from build123d import *

# Parameters (mm, degrees)
SKETCH_1_R          = 2.05
SKETCH_1_R_2        = 11.5
SKETCH_1_R_3        = 1.5
SKETCH_1_R_4        = 7.02
SKETCH_1_W          = 2.1
SKETCH_1_H          = 8.1
EXTRUDE_1_DEPTH     = 2
SKETCH_2_R          = 2
CUT_EXTRUDE_1_DEPTH = 4
FILLET_1_R          = 2


with BuildPart() as part:
    # 草图1 → 凸台-拉伸1 (new body)
    with BuildSketch(Plane.XY):
        with BuildLine():
            Line((-4.357142857, -0.045714286), (-4.357142857, 41.804285714))
            Line((-4.357142857, 41.804285714), (8.642857143, 41.804285714))
            Line((8.642857143, 41.804285714), (8.642857143, 14.954285714))
            Line((8.642857143, 14.954285714), (17.642857143, 14.954285714))
            Line((17.642857143, 14.954285714), (17.642857143, 41.804285714))
            Line((17.642857143, 41.804285714), (200.642857143, 41.804285714))
            Line((200.642857143, 41.804285714), (231.642857143, 30.954285714))
            ThreePointArc((231.642857143, 30.954285714), (262.642857143, -0.045714286), (231.642857143, -31.045714286))
            Line((231.642857143, -31.045714286), (200.656073527, -36.45591431))
            Line((200.656073527, -36.45591431), (193.846868021, -38.045714286))
            Line((193.846868021, -38.045714286), (22.465844759, -38.045714286))
            Line((22.465844759, -38.045714286), (3.792857143, -38.195714286))
            Line((3.792857143, -38.195714286), (3.792857143, -35.702553436))
            Line((3.792857143, -35.702553436), (-4.357142857, -35.702553436))
            Line((-4.357142857, -35.702553436), (-4.357142857, -0.045714286))
        make_face()
        with Locations((1.642857143, 29.954285714)):
            Circle(SKETCH_1_R, mode=Mode.SUBTRACT)
        with Locations((1.642857143, -0.045714286)):
            Circle(SKETCH_1_R, mode=Mode.SUBTRACT)
        with Locations((1.642857143, -30.045714286)):
            Circle(SKETCH_1_R, mode=Mode.SUBTRACT)
        with Locations((51.642857143, -0.045714286)):
            Circle(SKETCH_1_R_2, mode=Mode.SUBTRACT)
        with Locations((51.642857143, -14.045714286)):
            Circle(SKETCH_1_R_3, mode=Mode.SUBTRACT)
        with Locations((37.642857143, -0.045714286)):
            Circle(SKETCH_1_R_3, mode=Mode.SUBTRACT)
        with Locations((51.642857143, 13.954285714)):
            Circle(SKETCH_1_R_3, mode=Mode.SUBTRACT)
        with Locations((65.642857143, -0.045714286)):
            Circle(SKETCH_1_R_3, mode=Mode.SUBTRACT)
        with Locations((231.642857143, -0.045714286)):
            Circle(SKETCH_1_R_4, mode=Mode.SUBTRACT)
        with Locations((1.642857143, 14.954285714)):
            Rectangle(SKETCH_1_W, SKETCH_1_H, mode=Mode.SUBTRACT)
        with Locations((1.642857143, -15.045714286)):
            Rectangle(SKETCH_1_W, SKETCH_1_H, mode=Mode.SUBTRACT)
    extrude(amount=EXTRUDE_1_DEPTH)

    # 草图2 → 切除-拉伸1 (cut)
    with BuildSketch(Plane.XY.offset(2)):
        with Locations((26.642857143, 35.754285714)):
            Circle(SKETCH_2_R)
        with Locations((111.642857143, 35.754285714)):
            Circle(SKETCH_2_R)
        with Locations((196.642857143, 35.754285714)):
            Circle(SKETCH_2_R)
        with Locations((111.642857143, -34.245714286)):
            Circle(SKETCH_2_R)
        with Locations((196.642857143, -34.245714286)):
            Circle(SKETCH_2_R)
        with Locations((26.642857143, -34.245714286)):
            Circle(SKETCH_2_R)
        Polygon((187.542857143, -24.245714286), (140.41622539, -24.245714286), (187.542857143, 14.56445304), align=None)
        Polygon((122.542857143, 25.754285714), (169.669488896, 25.754285714), (122.542857143, -13.055881612), align=None)
        with BuildLine():
            Line((72.808867631, 8.954285714), (102.642857143, 8.954285714))
            Line((102.642857143, 8.954285714), (102.642857143, 26.754285714))
            Line((102.642857143, 26.754285714), (50.657939371, 26.754285714))
            Line((50.657939371, 26.754285714), (55.363054959, 22.651424922))
            ThreePointArc((55.363054959, 22.651424922), (65.846157695, 18.044787461), (72.808867631, 8.954285714))
        make_face()
        with BuildLine():
            Line((102.642857143, -9.045714286), (102.642857143, -26.845714286))
            Line((102.642857143, -26.845714286), (50.657939371, -26.845714286))
            Line((50.657939371, -26.845714286), (55.363054959, -22.742853493))
            ThreePointArc((55.363054959, -22.742853493), (65.846157695, -18.136216032), (72.808867631, -9.045714286))
            Line((72.808867631, -9.045714286), (102.642857143, -9.045714286))
        make_face()
        with BuildLine():
            Line((125.279005787, -19.870759717), (160.01586639, 8.736066661))
            ThreePointArc((160.01586639, 8.736066661), (163.433418031, 8.405335857), (163.102687227, 4.987784217))
            Line((163.102687227, 4.987784217), (128.365826624, -23.619042162))
            ThreePointArc((128.365826624, -23.619042162), (124.948274984, -23.288311358), (125.279005787, -19.870759717))
        make_face()
    extrude(amount=-CUT_EXTRUDE_1_DEPTH, mode=Mode.SUBTRACT)

    # 圆角1
    fillet_1_edges = [part.edges().sort_by_distance(p)[0] for p in [
        (72.808867631, 8.954285714, 1),
        (50.657939371, 26.754285714, 1),
        (102.642857143, 26.754285714, 1),
        (122.542857143, -13.055881612, 1),
        (122.542857143, 25.754285714, 1),
        (169.669488896, 25.754285714, 1),
        (187.542857143, 14.56445304, 1),
        (187.542857143, -24.245714286, 1),
        (140.41622539, -24.245714286, 1),
        (102.642857143, -26.845714286, 1),
        (50.657939371, -26.845714286, 1),
        (72.808867631, -9.045714286, 1),
        (102.642857143, -9.045714286, 1),
        (8.642857143, 41.804285714, 1),
        (17.642857143, 41.804285714, 1),
    ]]
    fillet(fillet_1_edges, radius=FILLET_1_R)


solid = part.part
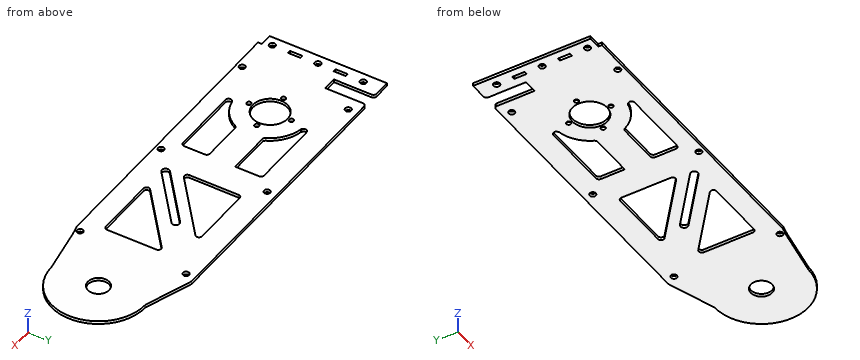
Part model, mm, in its own coordinate system. Give positions to 0.01 mm unless a question says otherwise; leave off trailing zeros. Loops run counter-clockwise (first coordinate to the right, second up) from the corner with the lowest first, then second, coordinate; pieces in that order, holes last.
(1) Band-saw the part on A-A (x = 177). Write the cut outline in (y, z), and give its area (3 significant figures).
Return value:
outline: (-38.05, 0) - (-24.25, 0) - (-24.25, 2) - (-38.05, 2) - close; (5.88, 0) - (41.8, 0) - (41.8, 2) - (5.88, 2) - close
area: 99.4 mm2
(2) Band-saw the part on B-B (z = 0.8). Count the separate pieces of the cut face and the enclosed holes in it, and give its area (3 significant figures).
Return value:
separate pieces: 1
enclosed holes: 22
area: 15,600 mm2
(3) Drill centre lines: line 1 along X through (y, z) = (-3.5, 1.35); line 2 along X through (y, z) = (-6, 0.35); line 3 along X through (y, z) = (13, 1.7). Where is each one in solid material? Low to high.
Return value:
line 1: x = -4.36 to 40.67, 62.61 to 122.54, 134.15 to 145.16, 152.8 to 165.61, 187.54 to 225.53, 237.75 to 262.45
line 2: x = -4.36 to 41.8, 61.48 to 122.54, 131.11 to 142.12, 149.76 to 162.57, 187.54 to 227.92, 235.36 to 262.07
line 3: x = -4.36 to 0.59, 2.69 to 50.49, 52.8 to 70.59, 102.64 to 122.54, 154.18 to 259.76
(4) Pin check, flat tips, straight feed: pin 1 (1 mm diameter, centred on x = 2, z = 1.5, fed in from -Y); pin 2 (5.5 mm diameter, centred on x = 1.64, y = -0.05, fed in from -Z); pin 3 (1 mm diameter, centred on y = 15.5, z = 1, fed in from +X); pin 4 (1 mm diameter, centred on y = 10.5, z = 1, fed in from +X). Stop position of each tip, or through.
Return value:
pin 1: stops at y = -35.7
pin 2: stops at z = 0
pin 3: stops at x = 258.75
pin 4: stops at x = 260.97
